The listing builds one solid part. Answer for the finished solid, in the listing's coordinates (mm). A direction names the side the tool comes from. Coordinates: 2 decimals unless noted, no trailing zeros. Write each loop counter-clockwise with the first axis right and the second up, starting at its lowest first coordinate (ties: lowest second). Pieces come first, ordered by that corner, then holes.
from build123d import *

# Parameters (mm, degrees)
SKETCH1_W               = 30
SKETCH1_H               = 20
BOSS_EXTRUDE1_DEPTH     = 8
SKETCH2_R               = 0.95
CUT_EXTRUDE1_DEPTH      = 20.723082923
BOSS_EXTRUDE2_START     = 2
SKETCH3_R               = 2
SKETCH3_R_2             = 0.95
BOSS_EXTRUDE2_DEPTH     = 2
CHAMFER1_SIZE           = 1.154700538
CHAMFER1_SIZE_2         = 2
SKETCH4_R               = 1.475
CUT_EXTRUDE2_DEPTH      = 21.615528128
LPATTERN1_COUNT         = 5
LPATTERN1_PITCH         = 5
LPATTERN1_COUNT_DIR2    = 2
LPATTERN1_PITCH_DIR2    = 5
MIRROR1_COPY_1_SKETCH_R = 1.475
MIRROR1_COPY_1_DEPTH    = 21.615528128
MIRROR1_COPY_2_SKETCH_R = 1.475
MIRROR1_COPY_2_DEPTH    = 21.615528128
MIRROR1_COPY_3_SKETCH_R = 1.475
MIRROR1_COPY_3_DEPTH    = 21.615528128
MIRROR1_COPY_4_SKETCH_R = 1.475
MIRROR1_COPY_4_DEPTH    = 21.615528128
MIRROR1_COPY_5_SKETCH_R = 1.475
MIRROR1_COPY_5_DEPTH    = 21.615528128
MIRROR1_COPY_6_SKETCH_R = 1.475
MIRROR1_COPY_6_DEPTH    = 21.615528128
MIRROR1_COPY_7_SKETCH_R = 1.475
MIRROR1_COPY_7_DEPTH    = 21.615528128
MIRROR1_COPY_8_SKETCH_R = 1.475
MIRROR1_COPY_8_DEPTH    = 21.615528128
SKETCH5_R               = 1.15
CUT_EXTRUDE3_DEPTH      = 2


with BuildPart() as part:
    # Sketch1 → Boss-Extrude1 (new body)
    with BuildSketch(Plane(origin=(0, 0, 0), x_dir=(1, 0, 0), z_dir=(0, 1, 0))):
        Rectangle(SKETCH1_W, SKETCH1_H)
    extrude(amount=BOSS_EXTRUDE1_DEPTH)

    # Sketch2 → Cut-Extrude1 (cut, through all)
    with BuildSketch(Plane(origin=(0, 8, 0), x_dir=(1, 0, 0), z_dir=(0, 1, 0))):
        with Locations(Location((-11.5, 7.75, 0), (0, 0, 270))):
            Circle(SKETCH2_R)
        with Locations(Location((-11.5, -7.75, 0), (0, 0, 270))):
            Circle(SKETCH2_R)
        with Locations(Location((11.5, -7.75, 0), (0, 0, 270))):
            Circle(SKETCH2_R)
        with Locations(Location((11.5, 7.75, 0), (0, 0, 270))):
            Circle(SKETCH2_R)
    extrude(amount=-CUT_EXTRUDE1_DEPTH, mode=Mode.SUBTRACT)

    # Sketch3 → Boss-Extrude2 (add)
    # profile 1 of 4: a face of its own
    with BuildSketch(Plane(origin=(0, 8, 0), x_dir=(1, 0, 0), z_dir=(0, 1, 0)).offset(BOSS_EXTRUDE2_START)):
        with Locations(Location((-11.5, -7.75, 0), (0, 0, 270))):
            Circle(SKETCH3_R)
        with Locations(Location((-11.5, -7.75, 0), (0, 0, 270))):
            Circle(SKETCH3_R_2, mode=Mode.SUBTRACT)
    # profile 2 of 4: a face of its own
    with BuildSketch(Plane(origin=(0, 8, 0), x_dir=(1, 0, 0), z_dir=(0, 1, 0)).offset(BOSS_EXTRUDE2_START)):
        with Locations(Location((-11.5, 7.75, 0), (0, 0, 270))):
            Circle(SKETCH3_R)
        with Locations(Location((-11.5, 7.75, 0), (0, 0, 270))):
            Circle(SKETCH3_R_2, mode=Mode.SUBTRACT)
    # profile 3 of 4: a face of its own
    with BuildSketch(Plane(origin=(0, 8, 0), x_dir=(1, 0, 0), z_dir=(0, 1, 0)).offset(BOSS_EXTRUDE2_START)):
        with Locations(Location((11.5, 7.75, 0), (0, 0, 270))):
            Circle(SKETCH3_R)
        with Locations(Location((11.5, 7.75, 0), (0, 0, 270))):
            Circle(SKETCH3_R_2, mode=Mode.SUBTRACT)
    # profile 4 of 4: a face of its own
    with BuildSketch(Plane(origin=(0, 8, 0), x_dir=(1, 0, 0), z_dir=(0, 1, 0)).offset(BOSS_EXTRUDE2_START)):
        with Locations(Location((11.5, -7.75, 0), (0, 0, 270))):
            Circle(SKETCH3_R)
        with Locations(Location((11.5, -7.75, 0), (0, 0, 270))):
            Circle(SKETCH3_R_2, mode=Mode.SUBTRACT)
    extrude(amount=-BOSS_EXTRUDE2_DEPTH)

    # Chamfer1
    # the kernel refuses this chamfer: 2, 1.154700538 mm, written as the material it adds along each edge
    with BuildSketch(Plane(origin=(11.5, 8, -7.75), x_dir=(0, 0, 1), z_dir=(-1, 0, 0))) as chamfer1_piece_1_section:
        Polygon((2 + CHAMFER1_SIZE, 0), (2, CHAMFER1_SIZE_2), (2, 0), align=None)
    chamfer1_piece_1 = revolve(axis=Axis((11.5, 8, -7.75), (0, 1, 0)), mode=Mode.PRIVATE)
    chamfer1_piece_1 = split(chamfer1_piece_1, bisect_by=Plane(origin=(14.074735909, 8.26258781, -10), z_dir=(0, 0, 1)), keep=Keep.TOP, mode=Mode.PRIVATE)
    chamfer1_piece_1 = split(chamfer1_piece_1, bisect_by=Plane(origin=(14.074735909, 10, -6.26347553), z_dir=(0, -1, 0)), keep=Keep.TOP, mode=Mode.PRIVATE)
    add(chamfer1_piece_1)
    with BuildSketch(Plane(origin=(11.5, 8, 7.75), x_dir=(0, 0, 1), z_dir=(-1, 0, 0))) as chamfer1_piece_2_section:
        Polygon((2 + CHAMFER1_SIZE, 0), (2, CHAMFER1_SIZE_2), (2, 0), align=None)
    chamfer1_piece_2 = revolve(axis=Axis((11.5, 8, 7.75), (0, 1, 0)), mode=Mode.PRIVATE)
    chamfer1_piece_2 = split(chamfer1_piece_2, bisect_by=Plane(origin=(11.5, 8.952348486, 10), z_dir=(0, 0, -1)), keep=Keep.TOP, mode=Mode.PRIVATE)
    chamfer1_piece_2 = split(chamfer1_piece_2, bisect_by=Plane(origin=(11.5, 10, 5.175184574), z_dir=(0, -1, 0)), keep=Keep.TOP, mode=Mode.PRIVATE)
    add(chamfer1_piece_2)
    with BuildSketch(Plane(origin=(-11.5, 8, -7.75), x_dir=(0, 0, 1), z_dir=(-1, 0, 0))) as chamfer1_piece_3_section:
        Polygon((2 + CHAMFER1_SIZE, 0), (2, CHAMFER1_SIZE_2), (2, 0), align=None)
    chamfer1_piece_3 = revolve(axis=Axis((-11.5, 8, -7.75), (0, 1, 0)), mode=Mode.PRIVATE)
    chamfer1_piece_3 = split(chamfer1_piece_3, bisect_by=Plane(origin=(-8.925264091, 8.26258781, -10), z_dir=(0, 0, 1)), keep=Keep.TOP, mode=Mode.PRIVATE)
    chamfer1_piece_3 = split(chamfer1_piece_3, bisect_by=Plane(origin=(-8.925264091, 10, -6.26347553), z_dir=(0, -1, 0)), keep=Keep.TOP, mode=Mode.PRIVATE)
    add(chamfer1_piece_3)
    with BuildSketch(Plane(origin=(-11.5, 8, 7.75), x_dir=(0, 0, 1), z_dir=(-1, 0, 0))) as chamfer1_piece_4_section:
        Polygon((2 + CHAMFER1_SIZE, 0), (2, CHAMFER1_SIZE_2), (2, 0), align=None)
    chamfer1_piece_4 = revolve(axis=Axis((-11.5, 8, 7.75), (0, 1, 0)), mode=Mode.PRIVATE)
    chamfer1_piece_4 = split(chamfer1_piece_4, bisect_by=Plane(origin=(-11.5, 8.952348486, 10), z_dir=(0, 0, -1)), keep=Keep.TOP, mode=Mode.PRIVATE)
    chamfer1_piece_4 = split(chamfer1_piece_4, bisect_by=Plane(origin=(-11.5, 10, 5.175184573), z_dir=(0, -1, 0)), keep=Keep.TOP, mode=Mode.PRIVATE)
    add(chamfer1_piece_4)

    # Sketch4 → Cut-Extrude2 (cut, through all)
    with BuildSketch(Plane.XZ):
        with Locations(Location((-10, 0, 0), (0, 0, 270))):
            Circle(SKETCH4_R)
    cut_extrude2 = extrude(amount=-CUT_EXTRUDE2_DEPTH, mode=Mode.SUBTRACT)

    # LPattern1: Cut-Extrude2 5 × 2, 2 skipped
    with Locations(*[(i * LPATTERN1_PITCH, 0, j * LPATTERN1_PITCH_DIR2) for i in range(LPATTERN1_COUNT) for j in range(LPATTERN1_COUNT_DIR2) if (i, j) not in ((0, 0), (0, 1), (4, 1))]):
        add(cut_extrude2, mode=Mode.SUBTRACT)

    # Mirror1 copy 1 sketch → Mirror1 copy 1 (cut, through all)
    with BuildSketch(Plane(origin=(5, 0, 0), x_dir=(1, 0, 0), z_dir=(0, -1, 0))):
        with Locations((-10, 0)):
            Circle(MIRROR1_COPY_1_SKETCH_R)
    extrude(amount=-MIRROR1_COPY_1_DEPTH, mode=Mode.SUBTRACT)

    # Mirror1 copy 2 sketch → Mirror1 copy 2 (cut, through all)
    with BuildSketch(Plane(origin=(5, 0, -5), x_dir=(1, 0, 0), z_dir=(0, -1, 0))):
        with Locations((-10, 0)):
            Circle(MIRROR1_COPY_2_SKETCH_R)
    extrude(amount=-MIRROR1_COPY_2_DEPTH, mode=Mode.SUBTRACT)

    # Mirror1 copy 3 sketch → Mirror1 copy 3 (cut, through all)
    with BuildSketch(Plane(origin=(10, 0, 0), x_dir=(1, 0, 0), z_dir=(0, -1, 0))):
        with Locations((-10, 0)):
            Circle(MIRROR1_COPY_3_SKETCH_R)
    extrude(amount=-MIRROR1_COPY_3_DEPTH, mode=Mode.SUBTRACT)

    # Mirror1 copy 4 sketch → Mirror1 copy 4 (cut, through all)
    with BuildSketch(Plane(origin=(10, 0, -5), x_dir=(1, 0, 0), z_dir=(0, -1, 0))):
        with Locations((-10, 0)):
            Circle(MIRROR1_COPY_4_SKETCH_R)
    extrude(amount=-MIRROR1_COPY_4_DEPTH, mode=Mode.SUBTRACT)

    # Mirror1 copy 5 sketch → Mirror1 copy 5 (cut, through all)
    with BuildSketch(Plane(origin=(15, 0, 0), x_dir=(1, 0, 0), z_dir=(0, -1, 0))):
        with Locations((-10, 0)):
            Circle(MIRROR1_COPY_5_SKETCH_R)
    extrude(amount=-MIRROR1_COPY_5_DEPTH, mode=Mode.SUBTRACT)

    # Mirror1 copy 6 sketch → Mirror1 copy 6 (cut, through all)
    with BuildSketch(Plane(origin=(15, 0, -5), x_dir=(1, 0, 0), z_dir=(0, -1, 0))):
        with Locations((-10, 0)):
            Circle(MIRROR1_COPY_6_SKETCH_R)
    extrude(amount=-MIRROR1_COPY_6_DEPTH, mode=Mode.SUBTRACT)

    # Mirror1 copy 7 sketch → Mirror1 copy 7 (cut, through all)
    with BuildSketch(Plane(origin=(20, 0, 0), x_dir=(1, 0, 0), z_dir=(0, -1, 0))):
        with Locations((-10, 0)):
            Circle(MIRROR1_COPY_7_SKETCH_R)
    extrude(amount=-MIRROR1_COPY_7_DEPTH, mode=Mode.SUBTRACT)

    # Mirror1 copy 8 sketch → Mirror1 copy 8 (cut, through all)
    with BuildSketch(Plane.XZ):
        with Locations((-10, 0)):
            Circle(MIRROR1_COPY_8_SKETCH_R)
    extrude(amount=-MIRROR1_COPY_8_DEPTH, mode=Mode.SUBTRACT)

    # Sketch5 → Cut-Extrude3 (cut)
    with BuildSketch(Plane(origin=(0, 10, 0), x_dir=(1, 0, 0), z_dir=(0, 1, 0))):
        with Locations(Location((-11.5, 7.75, 0), (0, 0, 270))):
            Circle(SKETCH5_R)
        with Locations(Location((-11.5, -7.75, 0), (0, 0, 270))):
            Circle(SKETCH5_R)
        with Locations(Location((11.5, 7.75, 0), (0, 0, 270))):
            Circle(SKETCH5_R)
        with Locations(Location((11.5, -7.75, 0), (0, 0, 270))):
            Circle(SKETCH5_R)
    extrude(amount=-CUT_EXTRUDE3_DEPTH, mode=Mode.SUBTRACT)


solid = part.part
Q1. The part is cut by section C-C, the plane z = -7.75. Write down the section's boundary in (x, y), then the cut area to 3 significant figures.
Answers below:
outline: (-15, 0) - (-12.45, 0) - (-12.45, 8) - (-12.65, 8) - (-12.65, 10) - (-13.5, 10) - (-14.65, 8) - (-15, 8) - close; (-10.55, 0) - (10.55, 0) - (10.55, 8) - (10.35, 8) - (10.35, 10) - (9.5, 10) - (8.35, 8) - (-8.35, 8) - (-9.5, 10) - (-10.35, 10) - (-10.35, 8) - (-10.55, 8) - close; (12.45, 0) - (15, 0) - (15, 8) - (14.65, 8) - (13.5, 10) - (12.65, 10) - (12.65, 8) - (12.45, 8) - close
area: 221 mm2
Q2. Which of the six approach directions +Z, -Z, +X, -X, +Y, -Y give full straight-line access (tool end or side, diameter ignored) to faces 1 (the face through (0, 8, -2)), 2 (the face through (11, 10, 9))?
Answers below:
face 1: +Y
face 2: +Z, -Z, +X, -X, +Y
Q3. The part is cut by section A-A, the plane z = 0. Write down the section's boundary in (x, y) (3 decimals), then the cut area to 3 significant figures.
Answers below:
outline: (-15, 0) - (-11.475, 0) - (-11.475, 8) - (-15, 8) - close; (-8.525, 0) - (-6.475, 0) - (-6.475, 8) - (-8.525, 8) - close; (-3.525, 0) - (-1.475, 0) - (-1.475, 8) - (-3.525, 8) - close; (1.475, 0) - (3.525, 0) - (3.525, 8) - (1.475, 8) - close; (6.475, 0) - (8.525, 0) - (8.525, 8) - (6.475, 8) - close; (11.475, 0) - (15, 0) - (15, 8) - (11.475, 8) - close
area: 122 mm2
Q4. Given pin 1 (6 mm diameter, centred on x = -3.5, z = 1.5, fed in from -Y); pin 2 (2 mm diameter, centred on x = -7, z = 0.5, fed in from +Y); pin 3 (1.8 mm diameter, centred on x = 11.5, z = -7.75, fed in from -Y), each flat-ended and moving along its own axis, determine where each tip first touches the part or whether it passes through.
Answers below:
pin 1: stops at y = 0
pin 2: stops at y = 8
pin 3: passes through
Q5. Determine the mould class of faces 3 (the face through (0, 4, 10)), 4 (the face through (0, 4, -10)), 5 (the face through (-0.192, 3.944, -3.538)) for opening direction Z: released by +Z, released by -Z, zero draft, split by the parting line, or undercut.
Answers below:
face 3: released by +Z
face 4: released by -Z
face 5: undercut
Q6. Find the intervals of material crossed by probe 1 along X at (y, z) = (3, -7.75); probe 2 along X at (y, z) = (5.75, 0) (3 decimals); probe 3 along Z at (x, y) = (10, 5.5) (3 decimals), in increasing order.
Answers below:
probe 1: x = -15 to -12.45, -10.55 to 10.55, 12.45 to 15
probe 2: x = -15 to -11.475, -8.525 to -6.475, -3.525 to -1.475, 1.475 to 3.525, 6.475 to 8.525, 11.475 to 15
probe 3: z = -10 to -1.475, 1.475 to 10
Q7. The part is cut by section D-D, the plane y = 6.25. State how many separate pieces and enclosed holes the cut face has, then the cut area to 3 significant figures.
Answers below:
separate pieces: 1
enclosed holes: 15
area: 513 mm2
Q8. The part is cut by section B-B, the plane x = 0. Write down the section's boundary in (y, z) (3 decimals).
Answers below:
outline: (0, -10) - (8, -10) - (8, -6.475) - (0, -6.475) - close; (0, -3.525) - (8, -3.525) - (8, -1.475) - (0, -1.475) - close; (0, 1.475) - (8, 1.475) - (8, 3.525) - (0, 3.525) - close; (0, 6.475) - (8, 6.475) - (8, 10) - (0, 10) - close
